The figure shows three views and two pictorial views of one solid part (mm, origin at its lowest corner). Answer the questions. A direction names the side the tool comes from. Coordinates: 2 decimals unless noted, no trailing zeros. Order: outer loops, then holes, each group sorted by start corner. A loop starts at its lowest first (then second) coordinate and runs counter-clockwise, first axis right, second up. Notation, with made-up numbers: M -39,-26 L 12,-26 A21 cw 12,0 Z; hole C 50,48.5 d6. An arc over 180 degrees is marked long. Answer in a Markdown table with one row per item. Add a question column.
Item 1: The part is cut by section C-C (z = 9). Write down the section's boundary in (x, y).
Item 2: Consider line 1 (Y direction, x = 18, z = 1.35); line 2 (Z direction, x = 7.5, y = 6.5); line 3 (Y direction, x = 17, z = 7.5). Determine where each line is inside the solid, lowest interval first. Write a range as from..to.
Item 3: The part is cut by section A-A (x = 18). Write down the section's boundary in (y, z), then the cut area to 3 significant figures.
Item 4: Flat-ended cylindrical pins translate along their axes: pin 1 Ø2.5 at (x, y) = (17.5, 34) entering from +Z; pin 2 Ø6 at (x, y) = (27, 9.5) entering from +Z; pin 3 Ø6 at (x, y) = (28, 7.5) entering from -Z; pin 4 Ø1.5 at (y, z) = (20.5, 9.5) entering from +X. Find the tip coordinate at first contact, or state that the pin passes through.
Item 5: Which of the six approach directions +Z, -Z, +X, -X, +Y, -Y give full straight-line access (tool end or side, diameter ignored) to the marked faces 1 and 2?
Item 6: The part is cut by section B-B (y = 18). Write down the section's boundary in (x, z), then the cut area to 3 significant figures.
Item 7: The mould has two halves that part along Y. Classify the marked faces 3, 4 and 5: released by +Y, released by -Y, zero draft, split by the parting line, or undercut.
Item 8: The part is cut by section D-D (x = 2.75). Write down the section's boundary in (y, z), then the cut area to 3 significant figures.
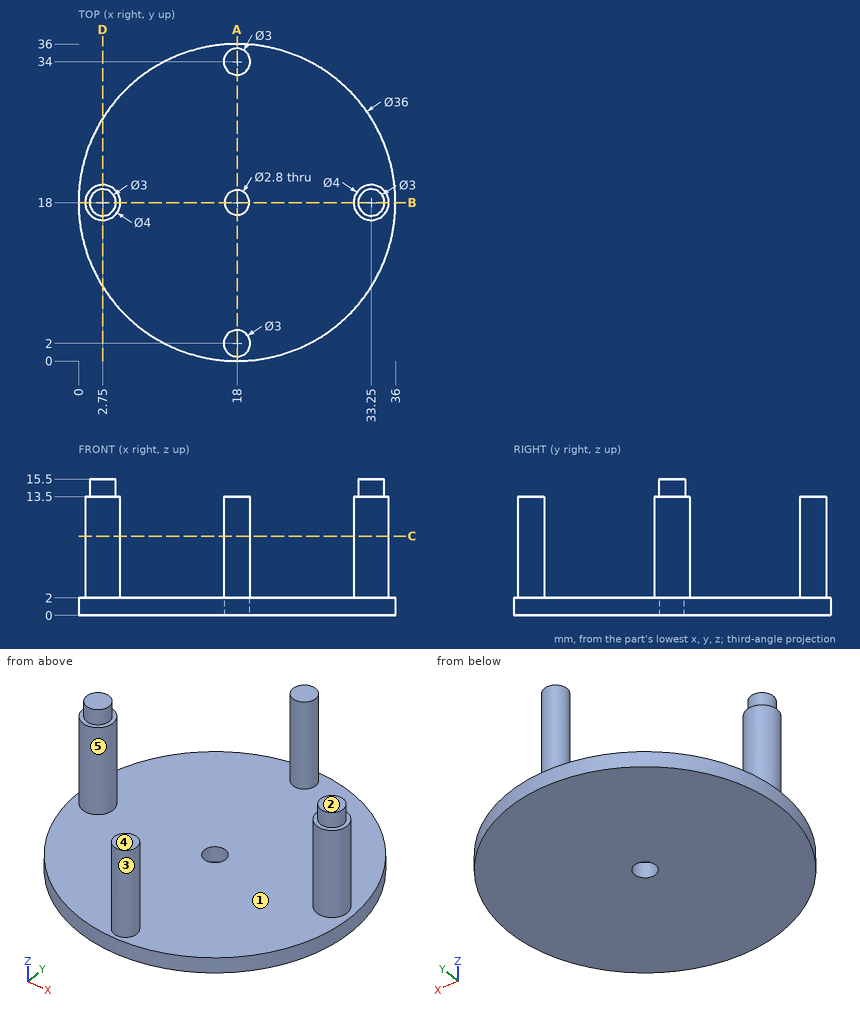
Reply:
| question | item | result |
|---|---|---|
| 1 | outline | C 2.75,18 d4; C 18,2 d3; C 18,34 d3; C 33.25,18 d4 |
| 2 | line 1 | y = 0..16.6, 19.4..36 |
| 2 | line 2 | z = 0..2 |
| 2 | line 3 | y = 0.88..3.12, 32.88..35.12 |
| 3 | outline | M 0,0 L 16.6,0 L 16.6,2 L 3.5,2 L 3.5,13.5 L 0.5,13.5 L 0.5,2 L 0,2 Z; M 19.4,0 L 36,0 L 36,2 L 35.5,2 L 35.5,13.5 L 32.5,13.5 L 32.5,2 L 19.4,2 Z |
| 3 | area | 135 mm2 |
| 4 | pin 1 | stops at z = 13.5 |
| 4 | pin 2 | stops at z = 2 |
| 4 | pin 3 | stops at z = 0 |
| 4 | pin 4 | stops at x = 34.22 |
| 5 | face 1 | +Z |
| 5 | face 2 | +Z, +X, -X, +Y, -Y |
| 6 | outline | M 0,0 L 16.6,0 L 16.6,2 L 4.75,2 L 4.75,13.5 L 4.25,13.5 L 4.25,15.5 L 1.25,15.5 L 1.25,13.5 L 0.75,13.5 L 0.75,2 L 0,2 Z; M 19.4,0 L 36,0 L 36,2 L 35.25,2 L 35.25,13.5 L 34.75,13.5 L 34.75,15.5 L 31.75,15.5 L 31.75,13.5 L 31.25,13.5 L 31.25,2 L 19.4,2 Z |
| 6 | area | 170 mm2 |
| 7 | face 3 | undercut |
| 7 | face 4 | zero draft |
| 7 | face 5 | split by the parting line |
| 8 | outline | M 8.44,0 L 27.56,0 L 27.56,2 L 20,2 L 20,13.5 L 19.5,13.5 L 19.5,15.5 L 16.5,15.5 L 16.5,13.5 L 16,13.5 L 16,2 L 8.44,2 Z |
| 8 | area | 90.2 mm2 |
